```python
from build123d import *

# Parameters (mm, degrees)
SKETCH006_W     = 9.5
SKETCH006_H     = 11.1
PAD004_DEPTH    = 4.4
PAD005_DEPTH    = 0.15
POCKET002_DEPTH = 0.25
SKETCH009_R     = 0.8
PAD006_DEPTH    = 0.4
FILLET003_R     = 0.2
SKETCH010_W     = 1
SKETCH010_H     = 0.6
PAD007_DEPTH    = 0.25
FILLET004_R     = 0.24
SKETCH011_W     = 0.75
SKETCH011_H     = 0.5
POCKET003_DEPTH = 9.5
FILLET005_R     = 0.5
POCKET004_DEPTH = 3.75
FILLET006_R     = 0.5
SKETCH013_W     = 3
SKETCH013_H     = 0.65
POCKET005_DEPTH = 0.2


with BuildPart() as part:
    # Sketch006 → Pad004 (new body)
    with BuildSketch(Plane.XZ):
        with Locations((0, -0.7)):
            Rectangle(SKETCH006_W, SKETCH006_H)
    extrude(amount=-PAD004_DEPTH)

    # Sketch007 (on Face6 of Pad004) → Pad005 (join)
    with BuildSketch(Plane(origin=(0, 4.4, 0), x_dir=(1, 0, 0), z_dir=(0, 1, 0))):
        with BuildLine():
            Line((-4.05, 2), (-4.05, -2))
            ThreePointArc((-4.05, -2), (-3.903553, -2.353553), (-3.55, -2.5))
            Line((-3.55, -2.5), (3.55, -2.5))
            ThreePointArc((3.55, -2.5), (3.903553, -2.353553), (4.05, -2))
            Line((4.05, -2), (4.05, 2))
            ThreePointArc((4.05, 2), (3.903553, 2.353553), (3.55, 2.5))
            Line((3.55, 2.5), (-3.55, 2.5))
            ThreePointArc((-3.55, 2.5), (-3.903553, 2.353553), (-4.05, 2))
        make_face()
    extrude(amount=PAD005_DEPTH)

    # Sketch008 (on Face5 of Pad005) → Pocket002 (cut)
    with BuildSketch(Plane(origin=(0, 4.4, 0), x_dir=(1, 0, 0), z_dir=(0, 1, 0))):
        with BuildLine():
            Line((-3.8, -2.7), (-4.75, -2.7))
            Line((-4.75, -2.7), (-4.75, -4.85))
            Line((-4.75, -4.85), (-2.85, -4.85))
            Line((-2.85, -4.85), (-2.85, -3.65))
            ThreePointArc((-2.85, -3.65), (-3.128249, -2.978249), (-3.8, -2.7))
        make_face()
        with BuildLine():
            Line((3.8, 4.6), (4.75, 4.6))
            Line((4.75, 4.6), (4.75, 2.7))
            Line((4.75, 2.7), (3.8, 2.7))
            ThreePointArc((3.8, 4.6), (2.85, 3.65), (3.8, 2.7))
        make_face()
    extrude(amount=-POCKET002_DEPTH, mode=Mode.SUBTRACT)

    # Sketch009 (on Face22 of Pocket002) → Pad006 (join)
    with BuildSketch(Plane(origin=(0, 4.15, 0), x_dir=(1, 0, 0), z_dir=(0, 1, 0))):
        with Locations((3.8, 3.65)):
            Circle(SKETCH009_R)
        with Locations((-3.8, -3.65)):
            Circle(SKETCH009_R)
    extrude(amount=PAD006_DEPTH)

    # Fillet003
    fillet003_edges = [part.edges().sort_by_distance(p)[0] for p in [
        (3, 4.55, -3.65),
        (-4.6, 4.55, 3.65),
    ]]
    fillet(fillet003_edges, radius=FILLET003_R)

    # Sketch010 (on Face12 of Fillet003) → Pad007 (join)
    with BuildSketch(Plane(origin=(0, 0, -6.25), x_dir=(1, 0, 0), z_dir=(0, 0, -1))):
        with Locations((-4.25, -0.8)):
            Rectangle(SKETCH010_W, SKETCH010_H)
        with Locations((-4.25, -4.1)):
            Rectangle(SKETCH010_W, SKETCH010_H)
        with Locations((4.25, -0.8)):
            Rectangle(SKETCH010_W, SKETCH010_H)
        with Locations((4.25, -4.1)):
            Rectangle(SKETCH010_W, SKETCH010_H)
    extrude(amount=PAD007_DEPTH)

    # Fillet004
    fillet004_edges = [part.edges().sort_by_distance(p)[0] for p in [
        (4.75, 4.1, -6.5),
        (4.75, 0.8, -6.5),
        (3.75, 0.8, -6.5),
        (3.75, 4.1, -6.5),
        (-3.75, 0.8, -6.5),
        (-4.75, 0.8, -6.5),
        (-3.75, 4.1, -6.5),
        (-4.75, 4.1, -6.5),
    ]]
    fillet(fillet004_edges, radius=FILLET004_R)

    # Sketch011 (on Face16 of Fillet004) → Pocket003 (cut)
    with BuildSketch(Plane(origin=(4.75, 0, 0), x_dir=(0, 0, 1), z_dir=(1, 0, 0))):
        with Locations((-5.875, -0.25)):
            Rectangle(SKETCH011_W, SKETCH011_H)
    extrude(amount=-POCKET003_DEPTH, mode=Mode.SUBTRACT)

    # Fillet005
    fillet005_edges = [part.edges().sort_by_distance(p)[0] for p in [
        (4.75, 2.45, -6.25),
        (-4.75, 2.45, -6.25),
    ]]
    fillet(fillet005_edges, radius=FILLET005_R)

    # Sketch012 (on Face22 of Fillet005) → Pocket004 (cut)
    with BuildSketch(Plane.XZ):
        with BuildLine():
            Line((3.75, 4.85), (3.75, 5.85))
            Line((3.75, 5.85), (5.75, 5.85))
            Line((5.75, 5.85), (5.75, 3.85))
            Line((5.75, 3.85), (4.75, 3.85))
            ThreePointArc((4.75, 3.85), (4.457107, 4.557107), (3.75, 4.85))
        make_face()
        with BuildLine():
            ThreePointArc((-3.75, 4.85), (-4.457107, 4.557107), (-4.75, 3.85))
            Line((-5.75, 3.85), (-4.75, 3.85))
            Line((-5.75, 5.85), (-5.75, 3.85))
            Line((-3.75, 5.85), (-5.75, 5.85))
            Line((-3.75, 4.85), (-3.75, 5.85))
        make_face()
    extrude(amount=-POCKET004_DEPTH, mode=Mode.SUBTRACT)

    # Fillet006
    fillet006_edges = [part.edges().sort_by_distance(p)[0] for p in [
        (4.75, 4.075, 4.85),
        (-4.75, 3.95, 4.85),
    ]]
    fillet(fillet006_edges, radius=FILLET006_R)

    # Sketch013 (on Face16 of Fillet006) → Pocket005 (cut)
    with BuildSketch(Plane(origin=(0, 0, 4.85), x_dir=(-1, 0, 0), z_dir=(0, 0, 1))):
        with Locations((0, -4.075)):
            Rectangle(SKETCH013_W, SKETCH013_H)
    extrude(amount=-POCKET005_DEPTH, mode=Mode.SUBTRACT)


solid = part.part
```
Work out the finished part from the listing and answer in its coordinate system (mm). A direction names the side the tool comes from. Coordinates: 2 decimals unless noted, no trailing zeros. Write each loop counter-clockwise with the first axis right and the second up, starting at its lowest first coordinate (ties: lowest second). Pieces come first, ordered by that corner, then holes.
Q1. A cutting plane is placed at C-C, the plane z = -3.65. Give the vertices of the cut face in (x, y), then the cut area to 3 significant figures.
Q2. Each of these flat-tipped pins is pushed along its axis until it touches: pin 1 Ø0.6 at (x, z) = (4, -6) entering from -Y; pin 2 Ø1 at (x, y) = (-0.5, 1) entering from -Z; pin 3 Ø5 at (x, z) = (2, 3.5) entering from +Y; pin 4 Ø0.6 at (x, y) = (-1.5, 0) entering from -Z. Where does it stop, or does it pass through?
Q3. Determine the mould class of faces 4 (the face through (-4.75, 2, -1)), 5 (the face through (0, 2, -6.25)), 6 (the face through (0, 0, 0)) for opening direction X: released by +X, released by -X, zero draft, split by the parting line, or undercut.
Q4. A cutting plane is placed at B-B, the plane x = 2.5. Give the vertices of the cut face in (y, z).
Q5. Which of the six approach directions +Z, -Z, +X, -X, +Y, -Y give full straight-line access (tool end or side, diameter ignored) to faces 1 (the face through (-4.449, 1.849, 4.565)), 2 (the face through (0, 4.4, -3)), 3 (the face through (0, 0.5, -6))?
Q6. Find the intervals of material crossed by line 1 (Z direction, x = -0.5, y = 1.05); line 2 (Y direction, x = -1.25, z = 3); line 3 (Z direction, x = 0, y = 3.8), in increasing order.
Q7. A cutting plane is placed at D-D, the plane z = -5. Give the vertices of the cut face in (x, y).
Q8. A cutting plane is placed at A-A, the plane y = 3.4. Give the vertices of the cut face in (x, z).
Findings below:
1. outline: (-4.75, 0) - (4.75, 0) - (4.75, 4.15) - (4.6, 4.15) - (4.6, 4.35) arc R0.2 ccw to (4.4, 4.55) - (3.2, 4.55) arc R0.2 ccw to (3, 4.35) - (3, 4.15) - (2.85, 4.15) - (2.85, 4.4) - (-4.75, 4.4) - close
1. area: 41.9 mm2
2. pin 1: stops at y = 0.5
2. pin 2: stops at z = -6.25
2. pin 3: stops at y = 4.55
2. pin 4: stops at z = -5.5
3. face 4: released by -X
3. face 5: undercut
3. face 6: zero draft
4. outline: (0, -5.5) - (0.5, -5.5) - (0.5, -6.25) - (4.4, -6.25) - (4.4, -2.5) - (4.55, -2.5) - (4.55, 2.5) - (4.4, 2.5) - (4.4, 4.85) - (0, 4.85) - close
5. face 1: +Z, -X, -Y
5. face 2: +Y
5. face 3: -Z, +X, -X, -Y
6. line 1: z = -6.25 to 4.85
6. line 2: y = 0 to 4.4
6. line 3: z = -6.25 to 4.65
7. outline: (-4.75, 0) - (4.75, 0) - (4.75, 4.4) - (-4.75, 4.4) - close
8. outline: (-4.75, -5.75) arc R0.5 ccw to (-4.25, -6.25) - (4.25, -6.25) arc R0.5 ccw to (4.75, -5.75) - (4.75, 3.85) arc R1 ccw to (3.75, 4.85) - (-3.75, 4.85) arc R1 ccw to (-4.75, 3.85) - close
